```python
from build123d import *

# Parameters (mm, degrees)
F0_W      = 89
F0_H      = 60
F0_W_2    = 85
F0_H_2    = 56
F1_DEPTH  = 10
F2_DEPTH  = 2
F3_W      = 13.3
F3_H      = 8.5
F3_W_2    = 16.5
F3_H_2    = 5
F4_DEPTH  = 18
F5_SIZE   = 0.75
F6_R      = 2.25
F6_R_2    = 1.25
F7_DEPTH  = 17.5
F8_DEPTH  = 13.5
F9_W      = 47.5
F9_H      = 40
F10_DEPTH = 25
F11_SIZE  = 9
F12_W     = 5
F12_H     = 6
F13_DEPTH = 2


with BuildPart() as f1:
    # F0 (on Top) → F1 (new body)
    with BuildSketch(Plane.XY):
        Rectangle(F0_W, F0_H)
        Rectangle(F0_W_2, F0_H_2, mode=Mode.SUBTRACT)
    extrude(amount=F1_DEPTH)

    # F0 (on Top) → F2 (join)
    with BuildSketch(Plane.XY):
        Rectangle(F0_W_2, F0_H_2)
    extrude(amount=F2_DEPTH)

    # F3 (on face) → F4 (cut)
    with BuildSketch(Plane.YZ.offset(44.5)):
        with Locations((-18.85, 5.75)):
            Rectangle(F3_W, F3_H)
        with Locations((-1.25, 5.75)):
            Rectangle(F3_W, F3_H)
        with Locations((17.35, 7.5)):
            Rectangle(F3_W_2, F3_H_2)
    extrude(amount=-F4_DEPTH, mode=Mode.SUBTRACT)

    # F5
    f5_edges = [f1.edges().sort_by_distance(p)[0] for p in [
        (44.5, 0, 0),
        (0, 30, 0),
        (-44.5, 0, 0),
        (0, -30, 0),
        (44.5, -30, 5),
        (-44.5, -30, 5),
        (-44.5, 30, 5),
        (44.5, 30, 5),
    ]]
    chamfer(f5_edges, length=F5_SIZE)

    # F6 (on face) → F7 (join)
    with BuildSketch(Plane.XY):
        with Locations((-39, -24.5)):
            Circle(F6_R)
        with Locations((-39, -24.5)):
            Circle(F6_R_2, mode=Mode.SUBTRACT)
        with Locations((19, -24.5)):
            Circle(F6_R)
        with Locations((19, -24.5)):
            Circle(F6_R_2, mode=Mode.SUBTRACT)
        with Locations((19, 24.5)):
            Circle(F6_R)
        with Locations((19, 24.5)):
            Circle(F6_R_2, mode=Mode.SUBTRACT)
        with Locations((-39, 24.5)):
            Circle(F6_R)
        with Locations((-39, 24.5)):
            Circle(F6_R_2, mode=Mode.SUBTRACT)
    extrude(amount=F7_DEPTH)

    # F8 (add): faces of the model
    f8_faces = [f1.faces().sort_by_distance(p)[0] for p in [
        (-39, 24.5, 2),
        (-39, -24.5, 2),
        (19, 24.5, 2),
        (19, -24.5, 2),
    ]]
    extrude(f8_faces, amount=F8_DEPTH)

    # F9 (on face) → F10 (cut)
    with BuildSketch(Plane.XY):
        with Locations((-10.75, 0)):
            Rectangle(F9_W, F9_H)
    extrude(amount=F10_DEPTH, mode=Mode.SUBTRACT)

    # F11
    f11_edges = [f1.edges().sort_by_distance(p)[0] for p in [
        (13, -20, 1),
        (-34.5, 20, 1),
    ]]
    chamfer(f11_edges, length=F11_SIZE)

    # F12 (on face) → F13 (cut)
    with BuildSketch(Plane.XZ.offset(30)):
        with Locations((34, 7)):
            Rectangle(F12_W, F12_H)
        with Locations((26, 7)):
            Rectangle(F12_W, F12_H)
        with Locations((18, 7)):
            Rectangle(F12_W, F12_H)
        with Locations((10, 7)):
            Rectangle(F12_W, F12_H)
        with Locations((2, 7)):
            Rectangle(F12_W, F12_H)
        with Locations((-6, 7)):
            Rectangle(F12_W, F12_H)
        with Locations((-14, 7)):
            Rectangle(F12_W, F12_H)
        with Locations((-22, 7)):
            Rectangle(F12_W, F12_H)
        with Locations((-30, 7)):
            Rectangle(F12_W, F12_H)
        with Locations((-38, 7)):
            Rectangle(F12_W, F12_H)
    extrude(amount=-F13_DEPTH, mode=Mode.SUBTRACT)


solid = f1.part
```
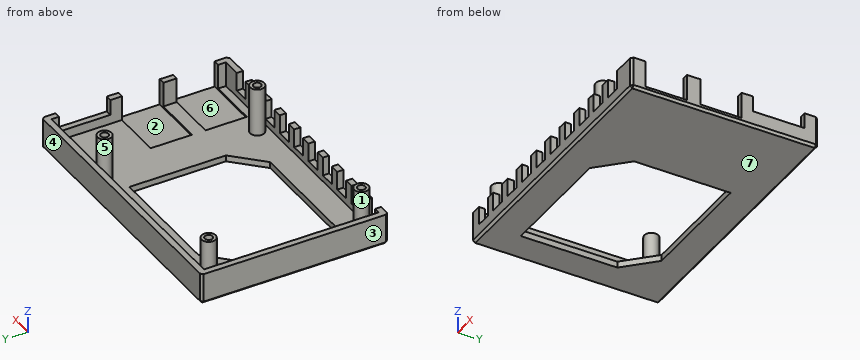
Model file for the job. Use its own axes, mm. Face numbers are marked on the shaded views. A direction names the side the tool comes from. Coordinates: 2 decimals unless noted, no trailing zeros. Loops run counter-clockwise (first coordinate to the right, second up) from the corner with the lowest first, then second, coordinate; pieces in that order, holes last. Notation, with made-up numbers: (-9, -35) - (17, -35) arc R8 ccw to (17, -25) - close; hole circle Ø1 at (82.5, 74). An arc over 180 degrees is marked (long way). Write item = value, one per line. Start each with the question number.
Item 1: Saw through at C-C, the plane y = -24.5. List the corners of the cut face in (x, z), then the cut area to 3 significant figures.
Item 2: Pull direction Y, two halves, no side cores. Call the marked faces 4, 5, 6 and 7: +Y half, -Y half, draft (parallel to the pull), parting line (faces both ways), or undercut.
Item 3: Wall check: probe 1 along Y at (x, z) = (19, 16.8); probe 2 along X at (y, z) = (-24.5, 16.2); probe 3 along Y at (x, z) = (3, 3.5). Give the ranges that are in metal, low to high. Write a range as [from, to].
Item 4: 3-axis set-ups, long thin cutter, end or side, ignore diameter. For the marked faces 1, 2 and 3: which of +Z, -Z, +X, -X, +Y, -Y reach the whole face in a straight line?
Item 5: Saw through at B-B, the plane x = -1.5. List the corners of the cut face in (y, z), then the cut area to 3 significant figures.
Item 6: Drop flat-ended pins along their axis: pin 1 Ø2 at (x, y) = (-9.5, -29) entering from +Z; pin 2 Ø0.6 at (x, y) = (-5, -28.5) entering from +Z; pin 3 Ø0.6 at (y, z) = (-21, 2) entering from +X; pin 4 Ø5 at (y, z) = (-11.5, 14) entering from +X. Give the stop position or say it passes through.
Item 7: Saw through at A-A, the plane y = -17.5. List the corners of the cut face in (x, z).
Item 8: Saw through at D-D, the plane z = 7.5. State how many separate pieces and enclosed holes the cut face has, then the cut area to 3 significant figures.
Answers:
q1.outline = (-44.5, 0.75) - (-43.75, 0) - (43.75, 0) - (44.5, 0.75) - (44.5, 1.5) - (26.5, 1.5) - (26.5, 2) - (21.25, 2) - (21.25, 17.5) - (20.25, 17.5) - (20.25, 15.5) - (17.75, 15.5) - (17.75, 17.5) - (16.75, 17.5) - (16.75, 2) - (-36.75, 2) - (-36.75, 17.5) - (-37.75, 17.5) - (-37.75, 15.5) - (-40.25, 15.5) - (-40.25, 17.5) - (-41.25, 17.5) - (-41.25, 2) - (-42.5, 2) - (-42.5, 10) - (-44.5, 10) - close
q1.area = 314 mm2
q2.face_4 = +Y half
q2.face_5 = undercut
q2.face_6 = undercut
q2.face_7 = draft
q3.probe_1 = [-26.75, -25.75], [-23.25, -22.25], [22.25, 23.25], [25.75, 26.75]
q3.probe_2 = [-41.25, -40.25], [-37.75, -36.75], [16.75, 17.75], [20.25, 21.25]
q3.probe_3 = [-30, -28], [28, 30]
q4.face_1 = +Z
q4.face_2 = +Z, +X
q4.face_3 = +Z, -Z, -X, +Y, -Y
q5.outline = (-30, 0.75) - (-29.25, 0) - (-20, 0) - (-20, 2) - (-28, 2) - (-28, 10) - (-30, 10) - close; (20, 0) - (29.25, 0) - (30, 0.75) - (30, 10) - (28, 10) - (28, 2) - (20, 2) - close
q5.area = 71.4 mm2
q6.pin_1 = 10
q6.pin_2 = 4
q6.pin_3 = 26.5
q6.pin_4 = through
q7.outline = (-44.5, 0.75) - (-43.75, 0) - (-34.5, 0) - (-34.5, 2) - (-42.5, 2) - (-42.5, 10) - (-44.5, 10) - close; (6.5, 0) - (43.75, 0) - (44.5, 0.75) - (44.5, 1.5) - (26.5, 1.5) - (26.5, 2) - (6.5, 2) - close
q8.separate_pieces = 17
q8.enclosed_holes = 0
q8.area = 456 mm2
